Check sheet for the modelled part. Datum: model origin and axes. Units: mm. Give positions to 0.01 mm unless a question says otherwise; leave off trailing zeros. Loops run counter-clockwise (first coordinate to the right, second up) from the corner with the lowest first, then second, coordinate; pieces in that order, holes last. Notation, with made-up numbers: (-31.75, 1) -> (15.25, 1) arc R22 ccw to (15.25, 23) -> close; hole circle Ø10 at (53.5, 66). An arc over 180 degrees is marked (long way). Answer as CSV lines item,"result". Start each with the question number.
(1) Material ranges on line 1 (Z direction, x = -430, y = 50); line 2 (Y direction, x = -544.5, z = -96.5); line 3 (X direction, y = 35, z = -108.5), recorded low to high. Write a range as from..to.
(2) Gauge pin test, flat ends, axial feed: pin 1 Ø6 at (x, z) = (-274, -87.5) entering from +Y; pin 2 Ø8 at (y, z) = (42, -93) entering from -X. Record the tip position at first contact, or that the pin passes through.
(3) Section check C-C on z = -92.5. Enter the section's corners in (x, y).
(4) Section check A-A on y = 72. Enter the section's corners in (x, z), plus the area to 3 significant figures.
(5) Section check B-B on x = -231.5. Enter the section's corners in (y, z), plus the area to 3 significant figures.
(6) Release check for a two-part mould opening along Z. For faces 1 (the face through (-55, 54, -109.22)), 2 (the face through (-12, 54, -5.08)), 3 (the face through (647.7, 50, -56)), 4 (the face through (-153, 52, -114.3)) record: pulls with the +Z half, pulls with the -Z half, needs draft (parallel to the pull), parting line crosses it, or undercut.
from build123d import *

# Parameters (mm, degrees)
SKETCH1_W           = 1295.4
SKETCH1_H           = 101.6
BOSS_EXTRUDE1_DEPTH = 114.3
SHELL1_T            = -5.08
SKETCH3_W           = 88.9
SKETCH3_H           = 96.52
CUT_EXTRUDE1_DEPTH  = 5.08


with BuildPart() as part:
    # Sketch1 → Boss-Extrude1 (new body)
    with BuildSketch(Plane.XY):
        with Locations((0, 50.8)):
            Rectangle(SKETCH1_W, SKETCH1_H)
    extrude(amount=-BOSS_EXTRUDE1_DEPTH)

    # Shell1
    shell1_openings = [part.faces().sort_by_distance(p)[0] for p in [
        (-647.7, 50.8, -57.15),
        (0, 101.6, -57.15),
    ]]
    offset(amount=SHELL1_T, openings=shell1_openings, kind=Kind.INTERSECTION)

    # Sketch3 → Cut-Extrude1 (cut)
    with BuildSketch(Plane(origin=(0, 0, -114.3), x_dir=(-1, 0, 0), z_dir=(0, 0, -1))):
        with Locations((-598.17, 53.34)):
            Rectangle(SKETCH3_W, SKETCH3_H)
    extrude(amount=-CUT_EXTRUDE1_DEPTH, mode=Mode.SUBTRACT)


solid = part.part
Working result:
1,line 1,"z = -114.3..-109.22, -5.08..0"
1,line 2,"y = 0..5.08"
1,line 3,"x = 642.62..647.7"
2,pin 1,"stops at y = 5.08"
2,pin 2,"stops at x = 642.62"
3,outline,"(-647.7, 0) -> (647.7, 0) -> (647.7, 101.6) -> (642.62, 101.6) -> (642.62, 5.08) -> (-647.7, 5.08) -> close"
4,outline,"(-647.7, -114.3) -> (553.72, -114.3) -> (553.72, -109.22) -> (-647.7, -109.22) -> close; (-647.7, -5.08) -> (642.62, -5.08) -> (642.62, -114.3) -> (647.7, -114.3) -> (647.7, 0) -> (-647.7, 0) -> close"
4,area,"13,200 mm^2"
5,outline,"(0, -114.3) -> (101.6, -114.3) -> (101.6, -109.22) -> (5.08, -109.22) -> (5.08, -5.08) -> (101.6, -5.08) -> (101.6, 0) -> (0, 0) -> close"
5,area,"1,560 mm^2"
6,face 1,"undercut"
6,face 2,"undercut"
6,face 3,"needs draft"
6,face 4,"pulls with the -Z half"
